```python
from build123d import *

# Parameters (mm, degrees)
SKETCH1_R           = 1.5
SKETCH1_R_2         = 1.75
SKETCH1_R_3         = 1.56
BOSS_EXTRUDE1_DEPTH = 3


with BuildPart() as part:
    # Sketch1 → Boss-Extrude1 (new body)
    with BuildSketch(Plane.XY):
        with BuildLine():
            Line((75, 50), (-75, 50))
            ThreePointArc((-75, 50), (-82.071067812, 47.071067812), (-85, 40))
            Line((-85, 40), (-85, -40))
            ThreePointArc((-85, -40), (-82.071067812, -47.071067812), (-75, -50))
            Line((-75, -50), (75, -50))
            ThreePointArc((75, -50), (82.071067812, -47.071067812), (85, -40))
            Line((85, -40), (85, -20))
            Line((85, -20), (85, 20))
            Line((85, 20), (85, 40))
            ThreePointArc((85, 40), (82.071067812, 47.071067812), (75, 50))
        make_face()
        with Locations((-75, -40)):
            Circle(SKETCH1_R, mode=Mode.SUBTRACT)
        with BuildLine():
            ThreePointArc((-71.5, -22.59), (-69.94, -24.15), (-71.5, -25.71))
            Line((-71.5, -25.71), (-74, -25.71))
            Line((-74, -25.71), (-76.5, -25.71))
            ThreePointArc((-76.5, -25.71), (-78.06, -24.15), (-76.5, -22.59))
            Line((-76.5, -22.59), (-74, -22.59))
            Line((-74, -22.59), (-71.5, -22.59))
        make_face(mode=Mode.SUBTRACT)
        with Locations((-75.5, -15)):
            Circle(SKETCH1_R_2, mode=Mode.SUBTRACT)
        with Locations((-51.5, -15)):
            Circle(SKETCH1_R_2, mode=Mode.SUBTRACT)
        with BuildLine():
            Line((25, -45.257829906), (-25, -45.257829906))
            ThreePointArc((-25, -45.257829906), (-29, -41.257829906), (-25, -37.257829906))
            Line((-25, -37.257829906), (25, -37.257829906))
            ThreePointArc((25, -37.257829906), (29, -41.257829906), (25, -45.257829906))
        make_face(mode=Mode.SUBTRACT)
        with Locations((19.9, -30)):
            Circle(SKETCH1_R_3, mode=Mode.SUBTRACT)
        with Locations((75, -40)):
            Circle(SKETCH1_R, mode=Mode.SUBTRACT)
        with Locations((74.9, -30)):
            Circle(SKETCH1_R_3, mode=Mode.SUBTRACT)
        with BuildLine():
            ThreePointArc((3.5, -22.59), (5.06, -24.15), (3.5, -25.71))
            Line((3.5, -25.71), (1, -25.71))
            Line((1, -25.71), (-1.5, -25.71))
            ThreePointArc((-1.5, -25.71), (-3.06, -24.15), (-1.5, -22.59))
            Line((-1.5, -22.59), (1, -22.59))
            Line((1, -22.59), (3.5, -22.59))
        make_face(mode=Mode.SUBTRACT)
        with Locations((0, -7.78)):
            Circle(SKETCH1_R_3, mode=Mode.SUBTRACT)
        with Locations((51.5, -15)):
            Circle(SKETCH1_R_2, mode=Mode.SUBTRACT)
        with Locations((75.5, -15)):
            Circle(SKETCH1_R_2, mode=Mode.SUBTRACT)
        with Locations((-75.5, 15)):
            Circle(SKETCH1_R_2, mode=Mode.SUBTRACT)
        with BuildLine():
            ThreePointArc((-72.5, 25.71), (-70.94, 24.15), (-72.5, 22.59))
            Line((-72.5, 22.59), (-75, 22.59))
            Line((-75, 22.59), (-77.5, 22.59))
            ThreePointArc((-77.5, 22.59), (-79.06, 24.15), (-77.5, 25.71))
            Line((-77.5, 25.71), (-75, 25.71))
            Line((-75, 25.71), (-72.5, 25.71))
        make_face(mode=Mode.SUBTRACT)
        with Locations((-51.5, 15)):
            Circle(SKETCH1_R_2, mode=Mode.SUBTRACT)
        with Locations((-75, 40)):
            Circle(SKETCH1_R, mode=Mode.SUBTRACT)
        with Locations((0, 7.78)):
            Circle(SKETCH1_R_3, mode=Mode.SUBTRACT)
        with BuildLine():
            ThreePointArc((10.05, 25.71), (11.61, 24.15), (10.05, 22.59))
            Line((10.05, 22.59), (7.55, 22.59))
            Line((7.55, 22.59), (5.05, 22.59))
            ThreePointArc((5.05, 22.59), (3.49, 24.15), (5.05, 25.71))
            Line((5.05, 25.71), (7.55, 25.71))
            Line((7.55, 25.71), (10.05, 25.71))
        make_face(mode=Mode.SUBTRACT)
        with Locations((51.5, 15)):
            Circle(SKETCH1_R_2, mode=Mode.SUBTRACT)
        with Locations((75.5, 15)):
            Circle(SKETCH1_R_2, mode=Mode.SUBTRACT)
        with Locations((19.9, 30)):
            Circle(SKETCH1_R_3, mode=Mode.SUBTRACT)
        with BuildLine():
            ThreePointArc((-25, 37.257829906), (-29, 41.257829906), (-25, 45.257829906))
            Line((-25, 45.257829906), (25, 45.257829906))
            ThreePointArc((25, 45.257829906), (29, 41.257829906), (25, 37.257829906))
            Line((25, 37.257829906), (-25, 37.257829906))
        make_face(mode=Mode.SUBTRACT)
        with Locations((74.9, 30)):
            Circle(SKETCH1_R_3, mode=Mode.SUBTRACT)
        with Locations((75, 40)):
            Circle(SKETCH1_R, mode=Mode.SUBTRACT)
    extrude(amount=BOSS_EXTRUDE1_DEPTH)


solid = part.part
```
The listing builds one solid part. Answer for the finished solid, in the listing's coordinates (mm). A direction names the side the tool comes from. Round coordinates to 2 decimals unless told otherwise and drop trailing zeros. Loops run counter-clockwise (first coordinate to the right, second up) from the corner with the lowest first, then second, coordinate; pieces in that order, holes last. Notation, with made-up numbers: (52, 29.5) - (77, 29.5) arc R25 cw to (77, 66.5) - close; hole circle Ø1 at (73.25, -27.75). An arc over 180 degrees is marked (long way). Return JSON: item names as keys, results as strings. Group by question number.
1. Consider probe 1 along Y at (x, z) = (-51.5, 1.55); probe 2 along Y at (x, z) = (18, 2.65); probe 3 along X at (y, z) = (8, 2.1). Determine where each line is inside the solid, lowest interval first.
2. The part is cut by section B-B on z = 2.5. State how many separate pieces and enclosed holes the cut face has, then the cut area to 3 significant figures.
3. This flat-tipped pin is pushed along its axis until it touches: P1, Ø5.5, axis at x = 75.5, y = -15, coming from the +Z side. Where does it stop, or does it pass through?
4. The part is cut by section C-C on x = -27. Determine the outline of the cut face in (y, z), then the cut area to 3 significant figures.
5. The part is cut by section A-A on x = 14.5. Determine the outline of the cut face in (y, z).
6. The mould has two halves that part along X. Classify faces 1 (the cylindrical face through (81.99, -47.15, 1.48)), 2 (the cylindrical face through (-81.99, 47.15, 1.48)), 3 (the cylindrical face through (-73.831, 15.526, 1.479)): pulls with the +X half, pulls with the -X half, needs draft (parallel to the pull), parting line crosses it, or undercut.
7. Which of the six approach directions +Z, -Z, +X, -X, +Y, -Y give full straight-line access (tool end or side, diameter ignored) to faces 4 (the flat face through (8, 25.71, 1)), 5 (the flat face through (1, 50, 1))?
Resolved:
{
 "1": {"probe 1": "y = -50 to -16.75, -13.25 to 13.25, 16.75 to 50", "probe 2": "y = -50 to -45.26, -37.26 to 37.26, 45.26 to 50", "probe 3": "x = -85 to -1.54, 1.54 to 85"},
 "2": {"separate pieces": "1", "enclosed holes": "24", "area": "15,800 mm²"},
 "3": {"P1": "stops at z = 3"},
 "4": {"outline": "(-50, 0) - (-44.72, 0) - (-44.72, 3) - (-50, 3) - close; (-37.79, 0) - (37.79, 0) - (37.79, 3) - (-37.79, 3) - close; (44.72, 0) - (50, 0) - (50, 3) - (44.72, 3) - close", "area": "258 mm²"},
 "5": {"outline": "(-50, 0) - (-45.26, 0) - (-45.26, 3) - (-50, 3) - close; (-37.26, 0) - (37.26, 0) - (37.26, 3) - (-37.26, 3) - close; (45.26, 0) - (50, 0) - (50, 3) - (45.26, 3) - close"},
 "6": {"face 1": "pulls with the +X half", "face 2": "pulls with the -X half", "face 3": "undercut"},
 "7": {"face 4": "+Z, -Z", "face 5": "+Z, -Z, +X, -X, +Y"}
}
